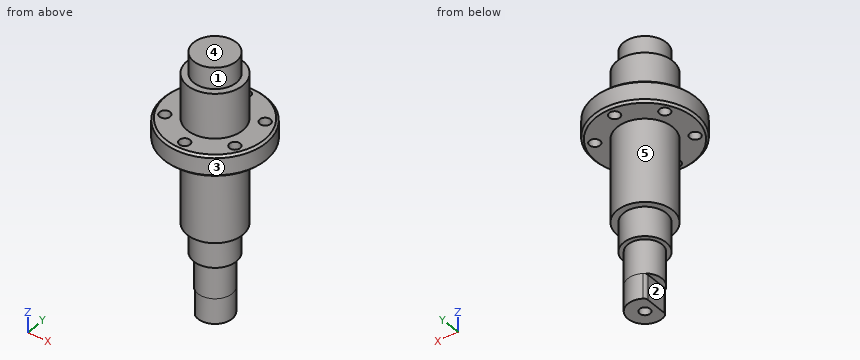
from build123d import *
from build123d.topology import SkipClean

# Parameters (mm, degrees)
HOLE_WIZARD_M3_1_D       = 2.5
PATTERN_CIRCULAR_1_COUNT = 6
CHAMFER_1_SIZE           = 0.5
SKETCH_5_OUTSIDE_W       = 38.908
SKETCH_5_OUTSIDE_H       = 38.908
SKETCH_5_OUTSIDE_R       = 4
CUT_EXTRUDE_1_DEPTH      = 8
EXTRUDE_START            = 5.9
EXTRUDE_1_DEPTH          = 5.9
HOLE_WIZARD_M3_2_D       = 2.5
HOLE_WIZARD_M3_2_DEPTH   = 7.5
HOLE_WIZARD_M3_2_TIP     = 0.751075774
FILLET_START             = -62
FILLET_1_DEPTH           = 7.1


with BuildPart() as part:
    # Sketch 1 → Revolve 1 (revolve)
    with BuildSketch(Plane(origin=(0, 0, 0), x_dir=(0, 0, -1), z_dir=(1, 0, 0))):
        Polygon((0, 0), (0, 5), (5, 5), (5, 6.5), (15.5, 6.5), (15.5, 12), (20.5, 12), (20.5, 6.5), (40, 6.5), (40, 5), (54.9, 5), (54.9, 0), align=None)
    revolve(axis=Axis((0, 0, -54.9), (0, 0, 1)))

    # Hole Wizard M3 _1 (through all)
    with Locations(Plane.XY.offset(-15.5)):
        with Locations((0, 9.5)):
            hole_wizard_m3_1 = Hole(HOLE_WIZARD_M3_1_D / 2)

    # Pattern Circular 1: Hole Wizard M3 _1 ×6 about axis
    pattern_circular_1_axis = Axis((0, 0, 0), (0, 0, 1))
    for i in range(1, PATTERN_CIRCULAR_1_COUNT):
        add(hole_wizard_m3_1.rotate(pattern_circular_1_axis, i * 360 / PATTERN_CIRCULAR_1_COUNT), mode=Mode.SUBTRACT)

    # Chamfer 1
    chamfer_1_edges = [part.edges().sort_by_distance(p)[0] for p in [
        (0, -12, -20.5),
        (0, -12, -15.5),
    ]]
    chamfer(chamfer_1_edges, length=CHAMFER_1_SIZE)

    # Sketch 5 outside → Cut-Extrude 1 (cut)
    with BuildSketch(Plane(origin=(0, 0, -54.9), x_dir=(-1, 0, 0), z_dir=(0, 0, -1))):
        Rectangle(SKETCH_5_OUTSIDE_W, SKETCH_5_OUTSIDE_H)
        with Locations(Location((0, 0, 0), (0, 0, 90))):
            Circle(SKETCH_5_OUTSIDE_R, mode=Mode.SUBTRACT)
    extrude(amount=-CUT_EXTRUDE_1_DEPTH, mode=Mode.SUBTRACT)

    # Sketch 6 → Extrude 1 (add)
    with SkipClean():  # the faces are left unmerged after this step: merging them gives an invalid solid
        with BuildSketch(Plane(origin=(0, 0, -54.9), x_dir=(-1, 0, 0), z_dir=(0, 0, -1)).offset(EXTRUDE_START)):
            with BuildLine():
                Line((2.6, 3.039736831), (2.6, -3.039736831))
                ThreePointArc((2.6, -3.039736831), (-4, 0), (2.6, 3.039736831))
            make_face()
        extrude(amount=-EXTRUDE_1_DEPTH)

    # Hole Wizard M3 _2
    with Locations(Plane(origin=(0, 0, -60.8), x_dir=(-1, 0, 0), z_dir=(0, 0, -1))):
        with Locations((0, 0)):
            Hole(HOLE_WIZARD_M3_2_D / 2, depth=HOLE_WIZARD_M3_2_DEPTH)
            with Locations((0, 0, -(HOLE_WIZARD_M3_2_DEPTH + HOLE_WIZARD_M3_2_TIP / 2))):  # 118° drill point
                Cone(0, HOLE_WIZARD_M3_2_D / 2, HOLE_WIZARD_M3_2_TIP, mode=Mode.SUBTRACT)

    # Fillet 1: read off the stored shape, not the designer's step
    # Fillet 1 outline → Fillet 1 (cut)
    with SkipClean():  # the faces are left unmerged after this step: merging them gives an invalid solid
        with BuildSketch(Plane.XY.offset(FILLET_START)):
            with BuildLine():
                ThreePointArc((-2.6, -3.039736831), (-2.372904367, -3.220143609), (-2.133333333, -3.383620677))
                ThreePointArc((-2.133333333, -3.383620677), (-2.475595036, -3.0207614), (-2.6, -2.537715508))
                Line((-2.6, -2.537715508), (-2.6, -3.039736831))
            make_face()
            with BuildLine():
                Line((-2.6, 3.039736831), (-2.6, 2.537715508))
                ThreePointArc((-2.6, 2.537715508), (-2.475595036, 3.0207614), (-2.133333333, 3.383620677))
                ThreePointArc((-2.133333333, 3.383620677), (-2.372904367, 3.220143609), (-2.6, 3.039736831))
            make_face()
        extrude(amount=FILLET_1_DEPTH, mode=Mode.SUBTRACT)


solid = part.part
Check sheet for the modelled part. Datum: model origin and axes. Units: mm. Face numbers are marked on the shaded views. A direction names the side the tool comes from. Give positions to 0.01 mm unless a question says otherwise; leave off trailing zeros. Order: outer loops, then holes, each group sorted by start corner. A loop starts at its lowest first (then second) coordinate and runs counter-clockwise, first axis right, second up. Notation, with made-up numbers: (54.25, -19) - (76.25, -19) arc R22 ccw to (76.25, -7) - close; hole circle Ø2 at (55.25, 56.5). An arc over 180 degrees is marked (long way). Answer as CSV lines item,"result".
1. Go/stop test with flat-tipped pins: P1, Ø2, axis at x = -8.23, y = -4.75, coming from the +Z side; P2, Ø10.5, axis at x = 0.5, y = 1.5, coming from the +Z side; P3, Ø5, axis at x = -6.5, y = -9, coming from the -Z side; P4, Ø3, axis at x = -9.5, z = -16, coming from the +Y side. Record where each tip stops, or that it passes through.
Result sheet:
P1,"through"
P2,"z = 0"
P3,"z = -20.5"
P4,"y = 8.94"
2. Section check A-A (z = -8). Record the boundary of the cut face in (x, y).
Result sheet:
outline,"circle Ø13 at (0, 0)"
3. Scan lines: probe 1 along Y at (x, z) = (0, -16.9); probe 2 along Y at (x, z) = (0, -57.75); probe 3 along Y at (x, z) = (-7.5, -19). Record each from-to range of solid material in increasing order. Write a range as from..to.
Result sheet:
probe 1,"-12..-10.75, -8.25..8.25, 10.75..12"
probe 2,"-4..-1.25, 1.25..4"
probe 3,"-9.37..-5.77, -3.73..3.73, 5.77..9.37"
4. Tool access check on the marked faces 1, 2, 3, 4 and 5. Record the directions out of +Z, -Z, +X, -X, +Y, -Y that give a thin tool (end or side, any length) a straight path to the whole face; none if there is none.
Result sheet:
face 1,"+Z"
face 2,"-Z, -X, +Y, -Y"
face 3,"+Z, -Z"
face 4,"+Z, +X, -X, +Y, -Y"
face 5,"-Z"
